Can you work these out from the model? Positions are in its coordinate system, mm. Face numbers are marked on the shaded views. A direction names the side the tool comes from. Coordinates: 2 decimals unless noted, no trailing zeros. Order: outer loops, then holes, each group sorted by start corner. A loop starts at its lowest first (then second) coordinate and runs counter-clockwise, first axis right, second up. Notation, with made-up numbers: (52, 9) - (60, 9) arc R22 cw to (60, 39) - close; hole circle Ø3 at (70, -36.5). An arc over 180 degrees is marked (long way). Return JSON: item names as keys, results as strings. Group by question number.
1) If I drill on line 1 along X through (y, z) = (-36.5, 13); line 2 along Z through (x, y) = (50.5, -10); line 3 along X through (y, z) = (-29.5, 15.5), over which ranges is the centre line in solid material (lowest first)?
2) For pin 1 Ø4 at (x, z) = (142, 11.5) entering from +Y; pin 2 Ø8.5 at (x, z) = (-4.5, 10) entering from -Y; pin 3 Ø12 at (x, z) = (121, 9) entering from -Y, each with a flat end and sliding along its axis, tell me the tip position at first contact or that it passes through.
3) Imagine slicing it at A-A (y = 8). Write out the boundary of the cut face in (x, z).
4) Which directions (+Z, -Z, +X, -X, +Y, -Y) give clear straight access to the entire face, cutting with the end or side of a thin tool? Please do the marked faces 1, 2 and 3.
5) Imagine slicing it at C-C (x = 93.5). Write out the boundary of the cut face in (y, z).
6) Imagine slicing it at D-D (y = 36). Write out the boundary of the cut face in (x, z).
```python
from build123d import *

# Parameters (mm, degrees)
BOSS_EXTRUDE1_DEPTH = 20
BOSS_EXTRUDE2_DEPTH = 5
FILLET1_R           = 15
FILLET2_R           = 10
FILLET3_R           = 15


# Some blends are built 0.0001 mm under size
with BuildPart() as part:
    # Sketch1 → Boss-Extrude1 (new body)
    with BuildSketch(Plane.XY):
        Polygon((0, 0), (0, -50), (15, -50), (15, 12.701705922), (177.765969889, 106.674682453), (170.265969889, 119.665063509), (-37.580127019, -0.334936491), (-47.580127019, 16.985571585), (-56.240381057, 11.985571585), (-32, -30), (-32, -50), (-17, -50), (-17, 0), align=None)
    extrude(amount=BOSS_EXTRUDE1_DEPTH)

    # Sketch2 → Boss-Extrude2 (add)
    with BuildSketch(Plane.XY):
        Polygon((15, -50), (143.985349671, 87.171432276), (15, 12.701705922), align=None)
    extrude(amount=BOSS_EXTRUDE2_DEPTH)

    # Fillet1
    # the kernel refuses this fillet: 15 mm, written as the material it takes off along each edge
    with BuildSketch(Plane(origin=(-56.240381057, 11.985571585, -35.355339059), x_dir=(0.866025403784439, 0.4999999999999994, 0), z_dir=(0, 0, 1))) as fillet1_piece_1:
        with BuildLine():
            CenterArc((15, -14.142135624), FILLET1_R, 109.471220634, 70.528779366)
            Line((0, -14.142135624), (-0.3, -14.142135624))
            Line((-0.3, -14.142135624), (-0.3, 0))
            Line((-0.3, 0), (0, 0.3))
            ThreePointArc((0, 0.3), (5, 0.3), (9.9, 0.282842712))
            Line((9.9, 0.282842712), (10, 0))
        make_face()
    extrude(amount=90.710678119, mode=Mode.SUBTRACT)

    # Fillet2
    fillet2_edges = [part.edges().sort_by_distance(p)[0] for p in [
        (-32, -50, 10),
    ]]
    fillet(fillet2_edges, radius=FILLET2_R)

    # Fillet3
    fillet3_edges = [part.edges().sort_by_distance(p)[0] for p in [
        (177.765969889, 106.674682453, 10),
    ]]
    fillet(fillet3_edges, radius=FILLET3_R - 0.0001)  # a hair under: the kernel refuses the full size


solid = part.part
```
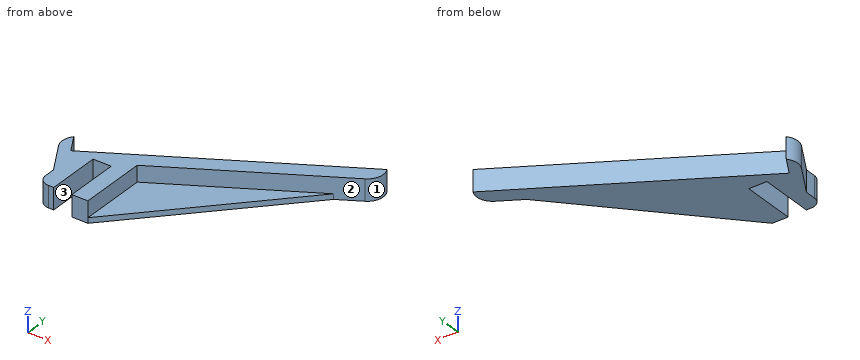
Calculated:
{
 "1": {"line 1": "-32 to -17, 0 to 15", "line 2": "0 to 5", "line 3": "-32.29 to -17, 0 to 15"},
 "2": {"pin 1": "y = 104.5", "pin 2": "y = 0", "pin 3": "y = 57.97"},
 "3": {"outline": "(-51.16, 0) - (-42.39, 0) - (-42.39, 20) - (-51.16, 20) - close; (-23.14, 0) - (69.54, 0) - (69.54, 5) - (15, 5) - (15, 20) - (-23.14, 20) - close"},
 "4": {"face 1": "+Z, -Z, +X", "face 2": "+Z, +X, -Y", "face 3": "+Z, -Z, -Y"},
 "5": {"outline": "(33.48, 0) - (75.34, 0) - (75.34, 20) - (58.02, 20) - (58.02, 5) - (33.48, 5) - close"},
 "6": {"outline": "(25.35, 0) - (95.87, 0) - (95.87, 5) - (55.35, 5) - (55.35, 20) - (25.35, 20) - close"}
}
